Answer from the drawing. Dimensions are ordinates in mm from the lowest x, y and z of the part. Coordinates: 2 decimals unless noted, no trailing zeros. Write each loop counter-clockwise with the first axis right and the second up, starting at its lowest first coordinate (ties: lowest second). Pieces come first, ordered by that corner, then holes. Notation, with made-up numbers: (45, 40) -> (53, 40) arc R12 cw to (53, 56) -> close; hole circle Ø2 at (-33.5, 84). An arc over 180 degrees is marked (long way). One line per item, written item: value. Start each with the question number.
1. Given P1, Ø3.5, axis at x = 18.5, y = 130.5, coming from the +Z side; P2, Ø6, axis at y = 59, z = 10, coming from the +X side; P3, Ø7.5, axis at x = 29.5, z = 41.5, coming from the -Y side; P4, Ø1, axis at x = 22, y = 41, coming from the +Z side, each flat-ended and moving along its own axis, determine where each tip first touches the part or whether it passes through.
2. Consider line 1 along Z through (x, y) = (3, 7); line 2 along X through (y, z) = (38.5, 38); line 3 along X through (y, z) = (77, 13.5). Determine where each line is inside the solid, lowest interval first.
3. Find section A-A, the plane y = 123.5. Write down the section's boundary in (x, z) (3 decimals).
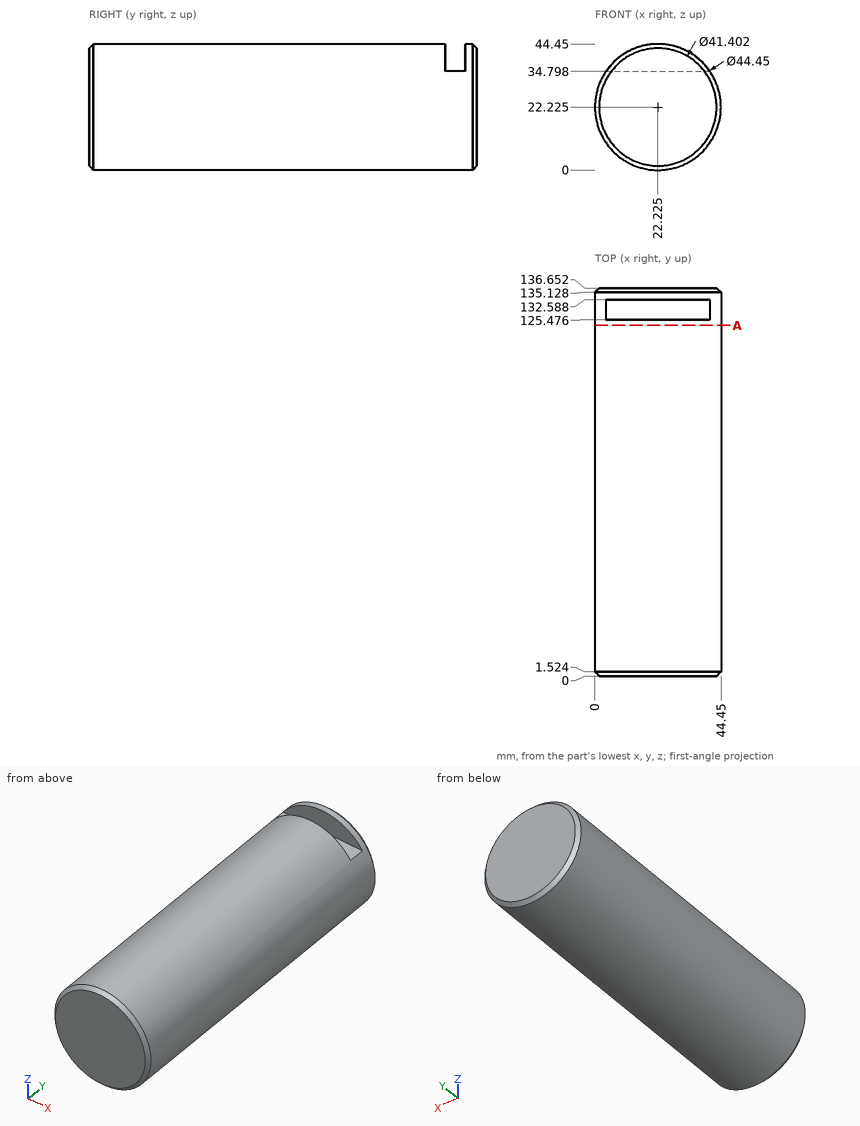
Answer block:
1. P1: stops at z = 34.8
1. P2: stops at x = 42.45
1. P3: stops at y = 0
1. P4: stops at z = 44.45
2. line 1: z = 11.07 to 33.38
2. line 2: x = 6.57 to 37.88
2. line 3: x = 1.78 to 42.67
3. outline: circle Ø44.45 at (22.225, 22.225)
